Read the model definition and answer for the solid it produces. Units are mm, in the model's axes. A direction names the side the tool comes from. Coordinates: 2 decimals unless noted, no trailing zeros. Loops run counter-clockwise (first coordinate to the right, second up) from the corner with the lowest first, then second, coordinate; pieces in that order, holes last. Notation, with made-up numbers: (26, 5.5) -> (67, 5.5) arc R19 cw to (67, 40.5) -> close; hole circle Ø1 at (11, -17). An arc over 180 degrees is marked (long way). Answer as a JSON object with one key per item and string values. Group by question number.
Q1. The part is cut by section C-C on x = -2.75. Write down the section's boundary in (y, z).
Q2. The part is cut by section B-B on y = -3. Write down the section's boundary in (x, z), and give its area (3 significant figures).
Q3. The part is cut by section D-D on y = 28.5. Write down the section's boundary in (x, z).
Q4. The part is cut by section A-A on z = 0. Write down the section's boundary in (x, y).
Q5. Each of these flat-tipped pins is pushed along its axis until it touches: P1, Ø5, axis at y = 27, z = -3.5, coming from the -X side; P2, Ø4, axis at x = -4, y = 20, coming from the +Z side. Where does it stop, or does it pass through?
Q6. For faces 5 (the flat face through (0, 0, 0)), 6 (the flat face through (3, -6.35, 0)), determine the directions among +Z, -Z, +X, -X, +Y, -Y from which every point of the face is accessible in a straight line to the end or side of a thin tool.
Q7. Straight lines are drawn through the part: line 1 along Y through (x, z) = (-2, 4.5); line 2 along Z through (x, y) = (1, 15); line 3 along X through (y, z) = (2, 3.5). For each, find the intervals that lie inside material, in ascending order. Write a range as [from, to].
Q8. Determine the mould class of faces 1 (the cylindrical face through (-0.651, 15.528, 4.957)), 2 (the cylindrical face through (4.31, -3.13, 0.38)), 3 (the cylindrical face through (-4.282, -3.131, -0.773)), 4 (the flat face through (-3, -6.35, 0)) for opening direction X: released by +X, released by -X, zero draft, split by the parting line, or undercut.
from build123d import *

# Parameters (mm, degrees)
F0_R     = 4.99999
F1_DEPTH = 31.496
F2_R     = 1.27
F3_DEPTH = 6.35


with BuildPart() as f1:
    # F0 (on Front) → F1 (new body)
    with BuildSketch(Plane.XZ):
        Circle(F0_R)
    extrude(amount=-F1_DEPTH)

    # F2 (on face) → F3 (join)
    with BuildSketch(Plane.XZ):
        with Locations((-3.274196, 0)):
            Circle(F2_R)
        with Locations((3.099181, 0)):
            Circle(F2_R)
    extrude(amount=F3_DEPTH)


solid = f1.part
Final values:
{
 "1": {"outline": "(-6.35, -1.16) -> (0, -1.16) -> (0, -4.18) -> (31.5, -4.18) -> (31.5, 4.18) -> (0, 4.18) -> (0, 1.16) -> (-6.35, 1.16) -> close"},
 "2": {"outline": "circle Ø2.54 at (-3.27, 0); circle Ø2.54 at (3.1, 0)", "area": "10.1 mm2"},
 "3": {"outline": "circle Ø10 at (0, 0)"},
 "4": {"outline": "(-5, 0) -> (-4.54, 0) -> (-4.54, -6.35) -> (-2, -6.35) -> (-2, 0) -> (1.83, 0) -> (1.83, -6.35) -> (4.37, -6.35) -> (4.37, 0) -> (5, 0) -> (5, 31.5) -> (-5, 31.5) -> close"},
 "5": {"P1": "stops at x = -4.9", "P2": "stops at z = 4.58"},
 "6": {"face 5": "-Y", "face 6": "+Z, -Z, +X, -X, -Y"},
 "7": {"line 1": "y = [0, 31.5]", "line 2": "z = [-4.9, 4.9]", "line 3": "x = [-3.57, 3.57]"},
 "8": {"face 1": "split by the parting line", "face 2": "undercut", "face 3": "undercut", "face 4": "zero draft"}
}
